```python
from build123d import *

# Parameters (mm, degrees)
SKETCH_1_R          = 6.5
EXTRUDE_192_DEPTH   = 13
SKETCH_2_R          = 3
CUT_EXTRUDE_1_DEPTH = 16.921683328
SKETCH_3_R          = 3.75
CUT_EXTRUDE_2_DEPTH = 8
CHAMFER_1_SIZE      = 0.5


with BuildPart() as part:
    # Эскиз1 → Extrude 192 (new body)
    with BuildSketch(Plane.XY):
        with Locations(Location((0, 0, 0), (0, 0, 180))):
            Circle(SKETCH_1_R)
    extrude(amount=EXTRUDE_192_DEPTH)

    # Эскиз2 → Вырез-Вытянуть1 (cut, through all)
    with BuildSketch(Plane.XY.offset(13)):
        Circle(SKETCH_2_R)
    extrude(amount=-CUT_EXTRUDE_1_DEPTH, mode=Mode.SUBTRACT)

    # Эскиз3 → Вырез-Вытянуть2 (cut)
    with BuildSketch(Plane.XY.offset(13)):
        Circle(SKETCH_3_R)
    extrude(amount=-CUT_EXTRUDE_2_DEPTH, mode=Mode.SUBTRACT)

    # Фаска1
    chamfer_1_edges = [part.edges().sort_by_distance(p)[0] for p in [
        (6.5, 0, 13),
    ]]
    chamfer(chamfer_1_edges, length=CHAMFER_1_SIZE)


solid = part.part
```
The listing builds one solid part. Answer for the finished solid, in the listing's coordinates (mm). A direction names the side the tool comes from. Round coordinates to 2 decimals unless told otherwise and drop trailing zeros. Loops run counter-clockwise (first coordinate to the right, second up) from the corner with the lowest first, then second, coordinate; pieces in that order, holes last. Notation, with made-up numbers: (71.5, 65) - (76.5, 65) arc R27 ccw to (76.5, 103) - close; hole circle Ø8 at (9, 64). An arc over 180 degrees is marked (long way). Use one line per item in the form item = value. Start each with the question number.
1. The part is cut by section D-D on z = 4. Determine the outline of the cut face in (x, y).
2. Consider line 1 (Y direction, x = 0, z = 1.65); line 2 (Y direction, x = 0, z = 10); line 3 (Z direction, x = 3, y = 2). Determine where each line is inside the solid, lowest interval first. Write a range as [from, to].
3. The part is cut by section A-A on x = 0. Determine the outline of the cut face in (y, z), then the cut area to 4 significant figures.
4. Given pin 1 Ø5 at (x, z) = (5, 10.5) entering from -Y; pin 2 Ø5 at (x, y) = (1, 0) entering from +Z; pin 3 Ø6 at (x, z) = (5, 3) entering from -Y, each flat-ended and moving along its own axis, determine where each tip first touches the part or whether it passes through.
5. A tool of negligible diameter and unlimited length cuts with its end or side. For faces 4 (the face through (-3.746, 0.165, 9.056)), 5 (the face through (-3, 1, 0)), from which of +Z, -Z, +X, -X, +Y, -Y can it reach the whole face along a straight path? Write none if from no direction.
6. The part is cut by section C-C on z = 8.25. Determine the outline of the cut face in (x, y).
7. For a pull along X with two mould halves and no side action, classify faces 1 (the face through (3, 3, 13)), 2 (the face through (5.158, 3.955, 6.162)), 3 (the face through (-3, 0, 3)) as pulls with the +X half, pulls with the -X half, needs draft (parallel to the pull), parting line crosses it, or undercut.
Geometry check:
q1.outline = circle Ø13 at (0, 0); hole circle Ø6 at (0, 0)
q2.line_1 = [-6.5, -3], [3, 6.5]
q2.line_2 = [-6.5, -3.75], [3.75, 6.5]
q2.line_3 = [0, 5]
q3.outline = (-6.5, 0) - (-3, 0) - (-3, 5) - (-3.75, 5) - (-3.75, 13) - (-6, 13) - (-6.5, 12.5) - close; (3, 0) - (6.5, 0) - (6.5, 12.5) - (6, 13) - (3.75, 13) - (3.75, 5) - (3, 5) - close
q3.area = 78.75 mm^2
q4.pin_1 = -6
q4.pin_2 = 5
q4.pin_3 = -6.18
q5.face_4 = +Z
q5.face_5 = -Z, +X, -X, +Y, -Y
q6.outline = circle Ø13 at (0, 0); hole circle Ø7.5 at (0, 0)
q7.face_1 = needs draft
q7.face_2 = parting line crosses it
q7.face_3 = undercut
